Geometry: see drawing. Coordinates: mm, zero at the bounding-box minimum. Give positions to 0.01 mm unless a question says otherwise; leave off trailing zeros. Order: outer loops, then holes, each group sorted by start corner. A loop starts at its lowest first (then second) coordinate and runs counter-clockwise, first axis right, second up. Notation, with made-up numbers: (29, -20) - (88, -20) arc R20 ccw to (88, 8) - close; hole circle Ø10 at (77.5, -29). An arc over 180 degrees is marked (long way). One line per item, written item: value.
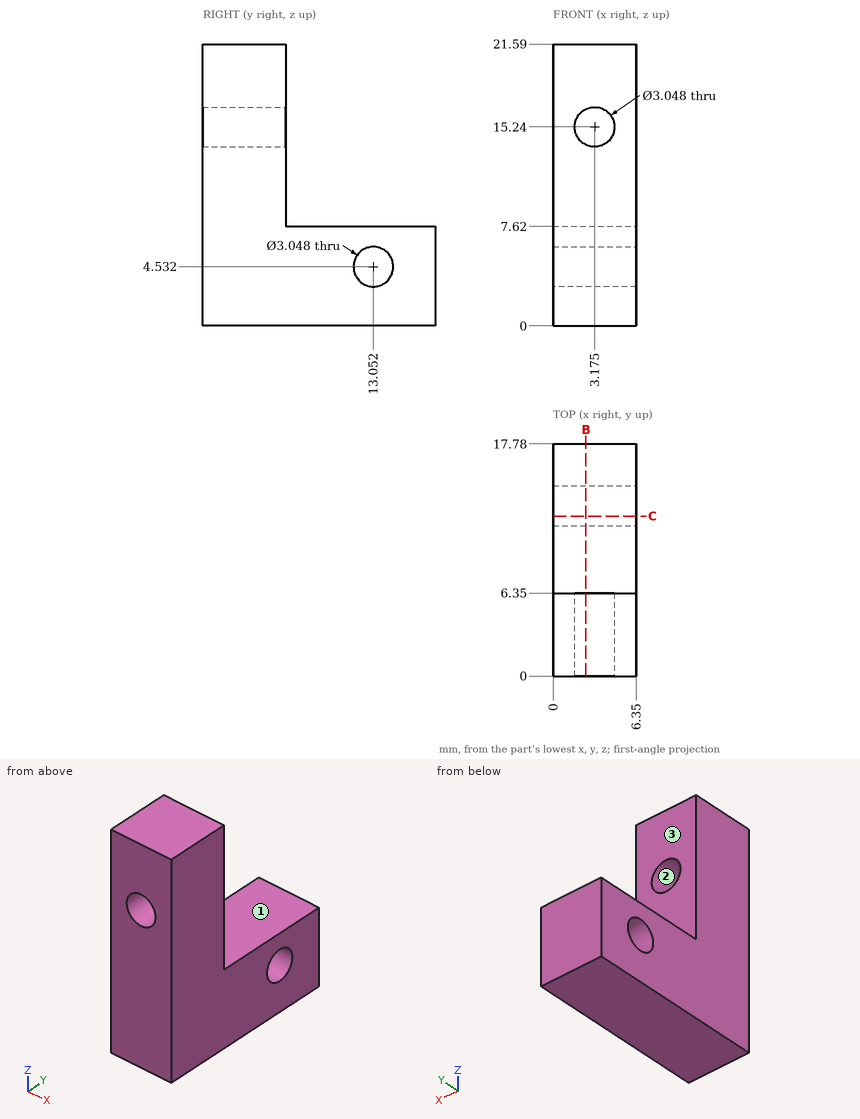
1) Material intervals for line 1 along Z through (x, y) = (2, 13) (1 decimal); line 2 along Y through (x, z) = (4.5, 4.5) (1 decimal); line 3 along Y through (x, z) = (2.75, 9), sorted ascending.
Answers below:
line 1: 0 to 3, 6.1 to 7.6
line 2: 0 to 11.5, 14.6 to 17.8
line 3: 0 to 6.35
2) Section C-C, the plane y = 12.25. Return loops of the section in (x, z).
Answers below:
outline: (0, 0) - (6.35, 0) - (6.35, 3.24) - (0, 3.24) - close; (0, 5.83) - (6.35, 5.83) - (6.35, 7.62) - (0, 7.62) - close
3) Section B-B, the plane x = 2.5. Return loops of the section in (y, z).
Answers below:
outline: (0, 0) - (17.78, 0) - (17.78, 7.62) - (6.35, 7.62) - (6.35, 13.87) - (0, 13.87) - close; (0, 16.61) - (6.35, 16.61) - (6.35, 21.59) - (0, 21.59) - close; hole circle Ø3.05 at (13.05, 4.53)
4) First-contact query: pin 1 (1 mm diameter, centred on x = 2.5, y = 10, fed in from +Z); pin 2 (2 mm diameter, centred on x = 1.5, z = 14.5, fed in from +Y). Flat tips, straight axial feed; report the tip coordinate or a pass-through.
Answers below:
pin 1: z = 7.62
pin 2: y = 6.35
5) Mould query, pull axis Z, two halves, no side actions, for the marked faces 1, 2 and 3. Classes: released by +Z, released by -Z, zero draft, split by the parting line, or undercut.
Answers below:
face 1: released by +Z
face 2: undercut
face 3: zero draft
